from build123d import *

# Parameters (mm, degrees)
SKETCH1_W           = 85
SKETCH1_H           = 95
BOSS_EXTRUDE1_DEPTH = 7
SKETCH2_W           = 35
SKETCH2_H           = 35
CUT_EXTRUDE1_DEPTH  = 7
CUT_EXTRUDE4_DEPTH  = 10
SKETCH12_W          = 85
SKETCH12_H          = 7
CUT_EXTRUDE9_DEPTH  = 0.5


with BuildPart() as part:
    # Sketch1 → Boss-Extrude1 (new body)
    with BuildSketch(Plane.XY):
        with Locations((42.5, 47.5)):
            Rectangle(SKETCH1_W, SKETCH1_H)
    extrude(amount=BOSS_EXTRUDE1_DEPTH)

    # Sketch2 → Cut-Extrude1 (cut)
    with BuildSketch(Plane.XY.offset(7)):
        with Locations((42.5, 45)):
            Rectangle(SKETCH2_W, SKETCH2_H)
    extrude(amount=-CUT_EXTRUDE1_DEPTH, mode=Mode.SUBTRACT)

    # Sketch7 → Cut-Extrude4 (cut)
    with BuildSketch(Plane(origin=(0, 0, 0), x_dir=(-1, 0, 0), z_dir=(0, 0, -1))):
        with BuildLine():
            Line((-85, 45), (-85, 0))
            Line((-85, 0), (0, 0))
            Line((0, 0), (0, 45))
            ThreePointArc((0, 45), (-42.5, 2.5), (-85, 45))
        make_face()
    extrude(amount=-CUT_EXTRUDE4_DEPTH, mode=Mode.SUBTRACT)

    # Sketch12 → Cut-Extrude9 (cut)
    with BuildSketch(Plane(origin=(0, 95, 0), x_dir=(1, 0, 0), z_dir=(0, 1, 0))):
        with Locations((42.5, -3.5)):
            Rectangle(SKETCH12_W, SKETCH12_H)
    extrude(amount=-CUT_EXTRUDE9_DEPTH, mode=Mode.SUBTRACT)


solid = part.part
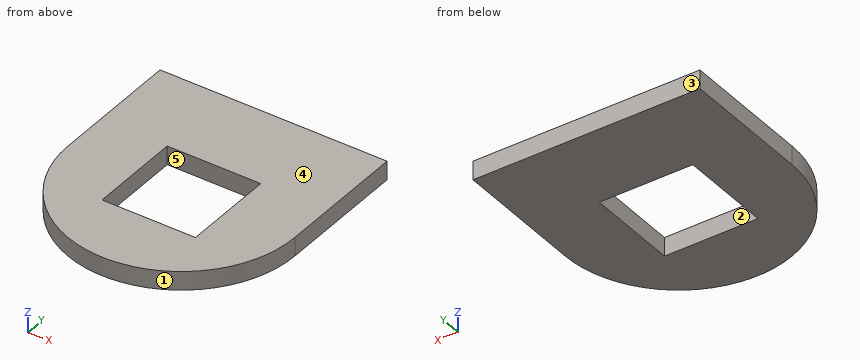
The model under review builds one solid part; all positions refer to its coordinate system, in mm. Face numbers are marked on the shaded views. A direction names the side the tool comes from. Give positions to 0.01 mm unless a question says otherwise; leave off trailing zeros. Loops run counter-clockwise (first coordinate to the right, second up) from the corner with the lowest first, then second, coordinate; pieces in that order, holes last. Notation, with made-up numbers: (83.5, 0.5) -> (130.5, 0.5) arc R28 cw to (130.5, 26.5) -> close; hole circle Ø2 at (-34.5, -8.5). An arc over 180 degrees is marked (long way). Put each result on its own line as item: value. Start each with the question number.
1. Clearance check with flat-ended pins moving along their axes: P1, Ø2, axis at y = 37, z = 5, coming from the -X side; P2, Ø2, axis at x = 74.5, y = 66, coming from the -Z side; P3, Ø2, axis at x = 34, z = 2, coming from the -Y side; P4, Ø1, axis at x = 16, z = 1, coming from the -Y side. State where each tip first meets the part, or that it passes through.
2. We need section A-A on x = 42.5. State the section outline as (y, z) points.
3. For the marked faces 4 and 5, list the 3-axis set-ups (+Z, -Z, +X, -X, +Y, -Y) from which the entire face can be reached by the end or side of a thin tool; tool diameter is ignored.
4. We need section C-C on x = 56. State the section outline as (y, z) points.
5. We need section B-B on z = 1.5. State the section outline as (x, y) points.
6. Wall thickness on probe 1 along X at (y, z) = (50, 3); probe 2 along Y at (x, z) = (43, 1.5); probe 3 along Y at (x, z) = (49, 3): over which ranges is each line inside the solid? List them lowest first.
7. We need section D-D on x = 80.5. State the section outline as (y, z) points, then the cut area to 3 significant figures.
8. Mouldability with a two-part tool opening along X and no side actions: class the marked faces 1, 2 and 3 as released by +X, released by -X, zero draft, split by the parting line, or undercut.
Determined:
1. P1: x = 0.58
1. P2: z = 0
1. P3: y = 3.17
1. P4: y = 11.38
2. outline: (2.5, 0) -> (27.5, 0) -> (27.5, 7) -> (2.5, 7) -> close; (62.5, 0) -> (94.5, 0) -> (94.5, 7) -> (62.5, 7) -> close
3. face 4: +Z, +X, -X, +Y, -Y
3. face 5: +Z, -Z
4. outline: (4.7, 0) -> (27.5, 0) -> (27.5, 7) -> (4.7, 7) -> close; (62.5, 0) -> (94.5, 0) -> (94.5, 7) -> (62.5, 7) -> close
5. outline: (0, 45) arc R42.5 ccw to (85, 45) -> (85, 94.5) -> (0, 94.5) -> close; hole (25, 27.5) -> (60, 27.5) -> (60, 62.5) -> (25, 62.5) -> close
6. probe 1: 0 to 25, 60 to 85
6. probe 2: 2.5 to 27.5, 62.5 to 94.5
6. probe 3: 3 to 27.5, 62.5 to 94.5
7. outline: (25.97, 0) -> (94.5, 0) -> (94.5, 7) -> (25.97, 7) -> close
7. area: 480 mm^2
8. face 1: split by the parting line
8. face 2: undercut
8. face 3: zero draft
